from build123d import *

# Parameters (mm, degrees)
BOSS_EXTRUDE1_DEPTH = 5
SKETCH2_R           = 3
SKETCH2_R_2         = 3.002001364
SKETCH2_R_3         = 2.999925667
SKETCH2_R_4         = 2.998527559
CUT_EXTRUDE2_DEPTH  = 5
SKETCH6_W           = 9.011632363
SKETCH6_H           = 16.045928836
SKETCH6_W_2         = 9.056347314
SKETCH6_H_2         = 16.054931831
CUT_EXTRUDE4_DEPTH  = 5
SKETCH8_R           = 1.49722604
SKETCH8_R_2         = 1.420293569
CUT_EXTRUDE6_DEPTH  = 5
SKETCH16_W          = 26.950881965
SKETCH16_H          = 4.917135509
CUT_EXTRUDE9_DEPTH  = 5
SKETCH11_R          = 1.497426658
SKETCH11_W          = 3.370796783
SKETCH11_H          = 16.122720009
CUT_EXTRUDE10_DEPTH = 10
SKETCH18_W          = 2.969435554
SKETCH18_H          = 16.028197631
CUT_EXTRUDE11_DEPTH = 10


with BuildPart() as part:
    # Sketch1 → Boss-Extrude1 (new body)
    with BuildSketch(Plane(origin=(0, 0, 0), x_dir=(1, 0, 0), z_dir=(0, 1, 0))):
        with BuildLine():
            Line((10, 0), (110, 0))
            ThreePointArc((110, 0), (117.071067812, -2.928932188), (120, -10))
            Line((120, -10), (120, -15))
            Line((120, -15), (115, -15))
            Line((115, -15), (115, -65))
            Line((115, -65), (120, -65))
            Line((120, -65), (120, -70))
            ThreePointArc((120, -70), (117.071067812, -77.071067812), (110, -80))
            Line((110, -80), (10, -80))
            ThreePointArc((10, -80), (2.928932188, -77.071067812), (0, -70))
            Line((0, -70), (0, -65))
            Line((0, -65), (5, -65))
            Line((5, -65), (5, -15))
            Line((5, -15), (0, -15))
            Line((0, -15), (0, -10))
            ThreePointArc((0, -10), (2.928932188, -2.928932188), (10, 0))
        make_face()
    extrude(amount=BOSS_EXTRUDE1_DEPTH)

    # Sketch2 → Cut-Extrude2 (cut)
    with BuildSketch(Plane(origin=(0, 5, 0), x_dir=(1, 0, 0), z_dir=(0, 1, 0))):
        with Locations((9.871405569, -8.58955783)):
            Circle(SKETCH2_R)
        with Locations((9.87978839, -71.481609293)):
            Circle(SKETCH2_R_2)
        with Locations((110.711521692, -71.131223036)):
            Circle(SKETCH2_R_3)
        with Locations((110.199519212, -8.625779617)):
            Circle(SKETCH2_R_4)
    extrude(amount=-CUT_EXTRUDE2_DEPTH, mode=Mode.SUBTRACT)

    # Sketch6 → Cut-Extrude4 (cut)
    with BuildSketch(Plane(origin=(0, 5, 0), x_dir=(1, 0, 0), z_dir=(0, 1, 0))):
        with Locations((20.155698208, -40.027815076)):
            Rectangle(SKETCH6_W, SKETCH6_H)
        with Locations((100.072460304, -40.013270259)):
            Rectangle(SKETCH6_W_2, SKETCH6_H_2)
    extrude(amount=-CUT_EXTRUDE4_DEPTH, mode=Mode.SUBTRACT)

    # Sketch8 → Cut-Extrude6 (cut)
    with BuildSketch(Plane(origin=(0, 5, 0), x_dir=(1, 0, 0), z_dir=(0, 1, 0))):
        with Locations((43.448740086, -34.53592606)):
            Circle(SKETCH8_R)
        with Locations((58.369614813, -34.660876222)):
            Circle(SKETCH8_R_2)
    extrude(amount=-CUT_EXTRUDE6_DEPTH, mode=Mode.SUBTRACT)

    # Sketch16 → Cut-Extrude9 (cut)
    with BuildSketch(Plane(origin=(0, 5, 0), x_dir=(1, 0, 0), z_dir=(0, 1, 0))):
        with Locations((51.607602958, -10.367487293)):
            Rectangle(SKETCH16_W, SKETCH16_H)
    extrude(amount=-CUT_EXTRUDE9_DEPTH, mode=Mode.SUBTRACT)

    # Sketch11 → Cut-Extrude10 (cut)
    with BuildSketch(Plane(origin=(0, 5, 0), x_dir=(1, 0, 0), z_dir=(0, 1, 0))):
        with Locations((10.104440234, -30.597351974)):
            Circle(SKETCH11_R)
        with Locations((10.104440234, -48.982097467)):
            Circle(SKETCH11_R)
        with Locations((109.853007641, -30.597351974)):
            Circle(SKETCH11_R)
        with Locations((109.853007641, -48.982097467)):
            Circle(SKETCH11_R)
        with Locations((93.839893868, -40.073898548)):
            Rectangle(SKETCH11_W, SKETCH11_H)
        with Locations((26.346912782, -40.066210662)):
            Rectangle(SKETCH11_W, SKETCH11_H)
    extrude(amount=-CUT_EXTRUDE10_DEPTH, mode=Mode.SUBTRACT)

    # Sketch18 → Cut-Extrude11 (cut)
    with BuildSketch(Plane(origin=(0, 5, 0), x_dir=(1, 0, 0), z_dir=(0, 1, 0))):
        with Locations((95.940490682, -40.026637359)):
            Rectangle(SKETCH18_W, SKETCH18_H)
    extrude(amount=-CUT_EXTRUDE11_DEPTH, mode=Mode.SUBTRACT)


solid = part.part
Can you work these out from the model? Positions are in its coordinate system, mm. A direction names the side the tool comes from. Coordinates: 2 decimals unless noted, no trailing zeros. Write each loop counter-clockwise with the first axis right and the second up, starting at its lowest first coordinate (ties: lowest second). Pieces come first, ordered by that corner, then holes. Notation, with made-up numbers: M -30.75,54 L 26.25,54 A18 cw 26.25,60 Z; hole C 43,76 d8. An arc over 180 degrees is marked long. Use one line per item in the form item = value.
Q1. For P1, Ø1.5, axis at y = 2.5, z = 39, coming from the -X side, with a flat end and sliding along its axis, tell me the tip position at first contact or that it passes through.
Model answer:
P1 = 5
Q2. If we section it at B-B (z = 46): Write out the boundary of the cut face in (x, y).
Model answer:
outline = M 5,0 L 15.65,0 L 15.65,5 L 5,5 Z; M 28.03,0 L 92.15,0 L 92.15,5 L 28.03,5 Z; M 104.6,0 L 115,0 L 115,5 L 104.6,5 Z
Q3. For faces 5 (the flat face through (94, 3, 32.013)), 6 (the flat face through (117, 2, 65)), 7 (the flat face through (61, 5, 39)), which set-ups out of +Z, -Z, +X, -X, +Y, -Y let a thin tool reach every point of the face, with its end or its side?
Model answer:
face_5 = +Y, -Y
face_6 = +X, +Y, -Y
face_7 = +Z, -Z, +X, -X, +Y
Q4. I need wall thicknesses on line 1 along Z through (x, y) = (58.5, 0.65); line 2 along Z through (x, y) = (28, 2.8); line 3 along Z through (x, y) = (108, 4.6). Which ranges of each line are inside material? Lowest first, please. Write a range as from..to.
Model answer:
line_1 = 0..7.91, 12.83..33.25, 36.08..80
line_2 = 0..32, 48.13..80
line_3 = 0..6.59, 10.66..69.85, 72.41..80
Q5. If we section it at C-C (x = 21.5): Write out the boundary of the cut face in (y, z), then the cut area to 3 significant figures.
Model answer:
outline = M 0,0 L 5,0 L 5,32 L 0,32 Z; M 0,48.05 L 5,48.05 L 5,80 L 0,80 Z
area = 320 mm^2
Q6. We'd pull the mould along Z, two halves only. Please class faces 1 (the cylindrical face through (42.261, 2.535, 35.447)), 2 (the flat face through (94, 3, 48.135)), 3 (the flat face through (120, 2, 12)), 4 (the flat face through (61, 2, 80)): +Z half, -Z half, draft (parallel to the pull), parting line (faces both ways), or undercut.
Model answer:
face_1 = undercut
face_2 = undercut
face_3 = draft
face_4 = +Z half
Q7. If we section it at A-A (x = 102): Write out the boundary of the cut face in (y, z).
Model answer:
outline = M 0,0 L 5,0 L 5,31.99 L 0,31.99 Z; M 0,48.04 L 5,48.04 L 5,80 L 0,80 Z
Q8. If we section it at D-D (y = 2.15): State how many separate pieces and enclosed holes the cut face has, then the cut area to 3 significant figures.
Model answer:
separate_pieces = 1
enclosed_holes = 13
area = 8,330 mm^2
